Autodesk Fusion 360 part; units mm, degrees
sketch "Skizze1" plane through (0, 0, 0) normal (0, 0, 1) x (1, 0, 0)
  line L0 (2.5, 11) -> (-2.5, 11)
  line L1 (-2.5, 11) -> (-2.5, -11)
  line L2 (-2.5, -11) -> (2.5, -11)
  line L3 (2.5, -11) -> (2.5, 11)
  line L4 (2.5, 11) -> (-2.5, -11) construction
  line L5 (-2.5, 11) -> (2.5, -11) construction
  line L6 (-2.5, -11) -> (2.5, -11)
  line L7 (2.5, -11) -> (2.5, -5)
  line L8 (2.5, -5) -> (-2.5, -5)
  line L9 (-2.5, -5) -> (-2.5, -11)
  line L10 (2.5, -5) -> (2.5, 5) construction
  line L11 (2.5, 5) -> (-2.5, 5)
  dimension "d1" = 5
  dimension "d2" = 22
  dimension "d3" = 5
  dimension "d4" = 6
  dimension "d13" = 10
extrude "Extrusion4" add sketch "Skizze1" along normal blind 3
extrude "Extrusion5" add sketch "Skizze1" along normal blind 5.2 contours L1 L2 L3 L6 L7 L8 L9
extrude "Extrusion6" cut sketch "Skizze1" along normal blind 1.25 contours L1 L3 L8 L11
Design review of the part built by this model. Coordinates are the model's own, in mm. A direction names the side the tool comes from. Give positions to 0.01 mm unless a question says otherwise; leave off trailing zeros. Write each loop counter-clockwise with the first axis right and the second up, starting at its lowest first coordinate (ties: lowest second). Pieces come first, ordered by that corner, then holes. Notation, with made-up numbers: M 26,41 L 35,41 A13 ccw 35,55 Z; hole C 20,34.5 d6. An arc over 180 degrees is marked long. Answer as a JSON object with one key per item and string values. Group by question number.
1) We need section C-C (y = 3.75). Give the boundary of the cut face in (x, z), and give its area (3 significant figures).
2) We need section B-B (x = -2.05). Give the boundary of the cut face in (y, z), and give its area (3 significant figures).
3) For line 1 along Y through (x, z) = (1.1, 4.4); line 2 along Z through (x, y) = (1.1, 3); line 3 along Z through (x, y) = (-0.7, 10), list the stretches that pass through material, from the lowest coordinate up.
4) We need section D-D (z = 3.2). Give the boundary of the cut face in (x, y), and give its area (3 significant figures).
5) We need section A-A (z = 0.4). Give the boundary of the cut face in (x, y), and give its area (3 significant figures).
6) Tool access review of faces 4 (the face through (0, -8, 0)), 5 (the face through (0, 5, 1)), 6 (the face through (0, 3, 3)): name each direction out of +Z, -Z, +X, -X, +Y, -Y from which nothing blocks a thin tool from reaching the whole face with its end or side.
7) Mouldability with a two-part tool opening along Y and no side actions: class faces 1 (the face through (0, 0, 1.25)), 2 (the face through (0, -5, 4)), 3 (the face through (0, -8, 5.2)) as released by +Y, released by -Y, zero draft, split by the parting line, or undercut.
8) Clearance check with flat-ended pins moving along their axes: pin 1 Ø2.5 at (x, y) = (0, 0.5) entering from -Z; pin 2 Ø2 at (x, y) = (1, 5.5) entering from +Z; pin 3 Ø2.5 at (x, z) = (0.5, 4.5) entering from +Y. State where each tip first meets the part, or that it passes through.
Answer key:
{
 "1": {"outline": "M -2.5,1.25 L 2.5,1.25 L 2.5,3 L -2.5,3 Z", "area": "8.75 mm²"},
 "2": {"outline": "M -11,0 L -5,0 L -5,1.25 L 5,1.25 L 5,0 L 11,0 L 11,3 L -5,3 L -5,5.2 L -11,5.2 Z", "area": "66.7 mm²"},
 "3": {"line 1": "y = -11 to -5", "line 2": "z = 1.25 to 3", "line 3": "z = 0 to 3"},
 "4": {"outline": "M -2.5,-11 L 2.5,-11 L 2.5,-5 L -2.5,-5 Z", "area": "30.0 mm²"},
 "5": {"outline": "M -2.5,-11 L 2.5,-11 L 2.5,-5 L -2.5,-5 Z; M -2.5,5 L 2.5,5 L 2.5,11 L -2.5,11 Z", "area": "60.0 mm²"},
 "6": {"face 4": "-Z, +X, -X, +Y, -Y", "face 5": "-Z, +X, -X", "face 6": "+Z, +X, -X, +Y"},
 "7": {"face 1": "undercut", "face 2": "released by +Y", "face 3": "zero draft"},
 "8": {"pin 1": "stops at z = 1.25", "pin 2": "stops at z = 3", "pin 3": "stops at y = -5"}
}
